The listing builds one solid part. Answer for the finished solid, in the listing's coordinates (mm). Face numbers are marked on the shaded views. A direction names the side the tool comes from. Coordinates: 2 decimals unless noted, no trailing zeros. Loops run counter-clockwise (first coordinate to the right, second up) from the corner with the lowest first, then second, coordinate; pieces in that order, holes last. Notation, with made-up numbers: (55, 41) - (88, 41) arc R28 ccw to (88, 79) - close; hole circle Ø6 at (-16.5, 2). An arc over 180 degrees is marked (long way). Put each result on its own line as item: value.
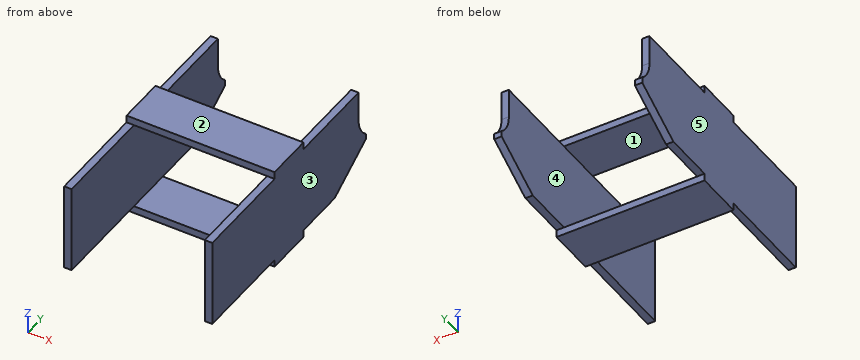
```python
from build123d import *

# Parameters (mm, degrees)
SKETCH_1_W          = 5
SKETCH_1_H          = 60
EXTRUDE_1_DEPTH     = 170
EXTRUDE_1_2_DEPTH   = 170
SKETCH_2_W          = 5
SKETCH_2_H          = 32
EXTRUDE_2_DEPTH     = 100
CUT_EXTRUDE_2_DEPTH = 120


with BuildPart() as part:
    # Sketch 1 → Extrude 1 (new body)
    with BuildSketch(Plane(origin=(0, 0, 0), x_dir=(1, 0, 0), z_dir=(0, 1, 0))):
        with Locations((-47.5, 0)):
            Rectangle(SKETCH_1_W, SKETCH_1_H)
    extrude(amount=EXTRUDE_1_DEPTH)



with BuildPart() as body_2:
    # Sketch 1 → Extrude 1 2 (new body)
    with BuildSketch(Plane(origin=(0, 0, 0), x_dir=(1, 0, 0), z_dir=(0, 1, 0))):
        with Locations((47.5, 0)):
            Rectangle(SKETCH_1_W, SKETCH_1_H)
    extrude(amount=EXTRUDE_1_2_DEPTH)


with BuildPart() as part_1:
    add(part.part)

    add(body_2.part)  # Extrude 2 merges body 2
    # Sketch 2 → Extrude 2 (add)
    with BuildSketch(Plane(origin=(50, 0, 0), x_dir=(0, 0, -1), z_dir=(1, 0, 0))):
        with Locations((-32.5, 85)):
            Rectangle(SKETCH_2_W, SKETCH_2_H)
        with Locations((32.5, 85)):
            Rectangle(SKETCH_2_W, SKETCH_2_H)
    extrude(amount=-EXTRUDE_2_DEPTH)

    # Sketch 3 → Cut-Extrude 2 (cut)
    with BuildSketch(Plane.ZY.offset(50)):
        Polygon((-10, 170), (-30, 135.5), (-48.568866089, 135.5), (-48.568866089, 174.591079236), (-10, 174.591079236), align=None)
        with BuildLine():
            Line((10, 162), (30, 162))
            Line((30, 162), (30, 182))
            ThreePointArc((30, 182), (-4.142135624, 196.142135624), (10, 162))
        make_face()
    extrude(amount=-CUT_EXTRUDE_2_DEPTH, mode=Mode.SUBTRACT)


solid = part_1.part
```
1) The part is cut by section B-B (z = -14). Give the vertices of the cut face in (x, y).
Found:
outline: (-50, 0) - (-45, 0) - (-45, 163.1) - (-50, 163.1) - close; (45, 0) - (50, 0) - (50, 163.1) - (45, 163.1) - close
2) For a pull along X with two mould halves and no side action, classify the marked faces 3, 4 and 5 as pulls with the +X half, pulls with the -X half, needs draft (parallel to the pull), parting line crosses it, or undercut.
Found:
face 3: pulls with the +X half
face 4: undercut
face 5: pulls with the -X half
3) For the marked faces 1 and 2, determine the directions among +Z, -Z, +X, -X, +Y, -Y from which every point of the face is accessible in a straight line to the end or side of a thin tool.
Found:
face 1: +Y, -Y
face 2: +Z, +X, -X, +Y, -Y
4) Each of these flat-tipped pins is pushed along its axis until it touches: pin 1 (10 mm diameter, centred on x = 25, y = 102, fed in from -Z); pin 2 (5.5 mm diameter, centred on x = -46.5, z = 21.5, fed in from +Y); pin 3 (1.5 mm diameter, centred on x = -48, y = 35.5, fed in from +Z); pin 4 (4 mm diameter, centred on x = -4.5, z = -33.5, fed in from -Y). Where does it stop, or does it pass through?
Found:
pin 1: stops at z = -35
pin 2: stops at y = 162
pin 3: stops at z = 30
pin 4: stops at y = 69
5) The part is cut by section A-A (x = 18.5). Give the vertices of the cut face in (y, z).
Found:
outline: (69, -35) - (101, -35) - (101, -30) - (69, -30) - close; (69, 30) - (101, 30) - (101, 35) - (69, 35) - close
6) Straight lines are drawn through the part: L1, parallel to X at y = 67, z = -10.5; L2, parallel to Z at x = 22, y = 87. For each, find the intervals that lie inside material, in ascending order. Write a range as [from, to].
Found:
L1: x = [-50, -45], [45, 50]
L2: z = [-35, -30], [30, 35]
7) The part is cut by section C-C (y = 78.5). Give the vertices of the cut face in (x, z), and give its area (3 significant figures).
Found:
outline: (-50, -35) - (50, -35) - (50, 35) - (-50, 35) - close; hole (-45, -30) - (45, -30) - (45, 30) - (-45, 30) - close
area: 1,600 mm^2
